```python
from build123d import *

# Parameters (mm, degrees)
SKETCH1_R           = 13
BOSS_EXTRUDE1_DEPTH = 5
FILLET1_R           = 5
FILLET2_R           = 3


with BuildPart() as part:
    # Sketch1 → Boss-Extrude1 (new, symmetric)
    with BuildSketch(Plane(origin=(0, 0, 0), x_dir=(1, 0, 0), z_dir=(0, 1, 0))):
        with BuildLine():
            Line((16.770509831, 5), (73.229490169, 5))
            ThreePointArc((73.229490169, 5), (107.5, 0), (73.229490169, -5))
            Line((73.229490169, -5), (16.770509831, -5))
            ThreePointArc((16.770509831, -5), (-17.5, 0), (16.770509831, 5))
        make_face()
        with Locations(Location((0, 0, 0), (0, 0, 270))):
            Circle(SKETCH1_R, mode=Mode.SUBTRACT)
        with Locations(Location((90, 0, 0), (0, 0, 270))):
            Circle(SKETCH1_R, mode=Mode.SUBTRACT)
    extrude(amount=BOSS_EXTRUDE1_DEPTH, both=True)

    # Fillet1
    fillet1_edges = [part.edges().sort_by_distance(p)[0] for p in [
        (16.770509831, 0, -5),
        (73.229490169, 0, -5),
        (73.229490169, 0, 5),
        (16.770509831, 0, 5),
    ]]
    fillet(fillet1_edges, radius=FILLET1_R)

    # Fillet2
    fillet2_edges = [part.edges().sort_by_distance(p)[0] for p in [
        (107.5, -5, 0),
        (107.5, 5, 0),
        (45, -5, 5),
        (45, 5, 5),
        (45, -5, -5),
        (45, 5, -5),
        (-17.5, -5, 0),
        (-17.5, 5, 0),
        (72.479587013, -5, 5.750817072),
        (72.479587013, 5, 5.750817072),
        (72.479587013, -5, -5.750817072),
        (72.479587013, 5, -5.750817072),
        (17.520412987, -5, -5.750817072),
        (17.520412987, 5, -5.750817072),
        (17.520412987, -5, 5.750817072),
        (17.520412987, 5, 5.750817072),
    ]]
    fillet(fillet2_edges, radius=FILLET2_R)


solid = part.part
```
Can you work these out from the model? Positions are in its coordinate system, mm. A direction names the side the tool comes from. Give positions to 0.01 mm unless a question says otherwise; leave off trailing zeros. Loops run counter-clockwise (first coordinate to the right, second up) from the corner with the lowest first, then second, coordinate; pieces in that order, holes last. Notation, with made-up numbers: M 54,38 L 88,38 A11 cw 88,43 Z; hole C 50.5,-32.75 d1. An arc over 180 degrees is marked long. One line per item, written item: value.
(1) Suppose I cut it at A-A on z = 0. List the corners of the cut face in (x, y) for me.
Returned:
outline: M -17.5,-2 A3 ccw -14.5,-5 L -13,-5 L -13,5 L -14.5,5 A3 ccw -17.5,2 Z; M 13,-5 L 77,-5 L 77,5 L 13,5 Z; M 103,-5 L 104.5,-5 A3 ccw 107.5,-2 L 107.5,2 A3 ccw 104.5,5 L 103,5 Z
(2) Suppose I cut it at B-B on x = 36.5. List the corners of the cut face in (y, z) for me, plus the area to 3 significant figures.
Returned:
outline: M -5,-2 A3 ccw -2,-5 L 2,-5 A3 ccw 5,-2 L 5,2 A3 ccw 2,5 L -2,5 A3 ccw -5,2 Z
area: 92.3 mm^2
(3) Suppose I cut it at C-C on z = 10. Count the separate pieces of the cut face and the enclosed holes in it, plus the area to 3 significant figures.
Returned:
separate pieces: 4
enclosed holes: 0
area: 223 mm^2
(4) Which directions (+Z, -Z, +X, -X, +Y, -Y) give clear straight access to the entire face, cutting with the end or side of a thin tool? Please do faces 1 (the face through (44.65, -4.14, 4.1)), 2 (the face through (45, 0, 5)), 3 (the face through (44.65, 4.14, 4.1)).
Returned:
face 1: +Z, -Y
face 2: +Z, +Y, -Y
face 3: +Z, +Y
(5) We'd pull the mould along X, two halves only. Please class faces 4 (the face through (45, 5, 0)), 5 (the face through (45.35, -4.14, -4.1)), 6 (the face through (107.488, 0.028, -0.657)): released by +X, released by -X, zero draft, split by the parting line, or undercut.
Returned:
face 4: zero draft
face 5: undercut
face 6: undercut
(6) Will these pins go through, and if not, where does the flat tip stop? pin 1 (4 mm diameter, centred on x = 28, z = -4.5, fed in from +Y); pin 2 (2 mm diameter, centred on x = 59, y = -2.5, fed in from -Z); pin 3 (6 mm diameter, centred on y = -1.5, z = 9, fed in from +X); pin 4 (12 mm diameter, centred on x = -1.5, z = 2, fed in from +Y).
Returned:
pin 1: y = 4.96
pin 2: z = -5
pin 3: x = 106.44
pin 4: through
(7) I need wall thicknesses on line 1 (X direction, y = -0.75, z = 0.5); line 2 (X direction, y = 1, z = -4); line 3 (X direction, y = 3, z = 7). Which ranges of each line are inside material? Lowest first, please.
Returned:
line 1: -17.49 to -12.99, 12.99 to 77.01, 102.99 to 107.49
line 2: -17.04 to -12.37, 12.37 to 77.63, 102.37 to 107.04
line 3: -15.85 to -10.95, 10.95 to 15.94, 74.06 to 79.05, 100.95 to 105.85
